Geometry: final body of the model. Coordinates: model frame, mm. A direction names the side the tool comes from. Round coordinates to 2 decimals unless told otherwise and drop trailing zeros. Loops run counter-clockwise (first coordinate to the right, second up) from the corner with the lowest first, then second, coordinate; pieces in that order, holes last. Notation, with made-up numbers: (49, 60.25) - (105, 60.25) arc R18 ccw to (105, 78.25) - close; hole circle Ø4 at (32.25, 41). An arc over 180 degrees is marked (long way). Answer as a JSON object with one key per item and string values. Group by question number.
Item 1: Section D-D (z = -8). Return the cut outline in (x, y).
Item 2: First-contact query: pin 1 (3 mm diameter, centred on y = 8.5, z = 16, fed in from +X); pin 2 (2 mm diameter, centred on x = 0.5, z = -2.5, fed in from -Y); pin 3 (2 mm diameter, centred on y = 15, z = -1, fed in from -X); pin 4 (4 mm diameter, centred on y = 4, z = 3.5, fed in from +X). Flat tips, straight axial feed; report the tip coordinate or a pass-through.
Item 3: Reachability of faces 1 (the face through (-10.06, 7.71, 16.31)), 2 (the face through (0, 0, 20.48)) from +Z, -Z, +X, -X, +Y, -Y: full face, straight path, thin tool, end or side. Return the list, or none.
Item 4: Line query: line 1 (Z direction, x = -17, y = 0.5); line 2 (Z direction, x = 8, y = -9); line 3 (X direction, y = -6, z = 5). Output: solid intervals per line, ascending.
Item 5: Draft query along Z for faces 3 (the face through (2.7, -14.2, -4.92)), 4 (the face through (-8.87, 6.8, 10.67)), 5 (the face through (-10.06, 7.71, 1.72)). Return one class per face: released by +Z, released by -Z, zero draft, split by the parting line, or undercut.
Item 6: Section C-C (z = 3). Return the cut outline in (x, y), plus the area to 3 significant figures.
```python
from build123d import *

# Parameters (mm, degrees)
F2_SIZE = 2.54
F3_R    = 1.5875


with BuildPart() as f1:
    # F0 (on Front) → F1 (revolve)
    with BuildSketch(Plane.XZ):
        with BuildLine():
            Line((12.6746, 20.479507), (0, 20.479507))
            Line((0, 20.479507), (0, -14.699493))
            Line((0, -14.699493), (19.05, -14.699493))
            Line((19.05, -14.699493), (19.05, -4.920493))
            Line((19.05, -4.920493), (14.2621, -4.920493))
            ThreePointArc((14.2621, -4.920493), (13.139568, -4.455525), (12.6746, -3.332993))
            Line((12.6746, -3.332993), (12.6746, 6.636507))
            Line((12.6746, 6.636507), (12.6746, 6.638998))
            ThreePointArc((12.6746, 6.638998), (11.609965, 7.133359), (11.176, 8.224007))
            Line((11.176, 8.224007), (11.176, 13.050007))
            ThreePointArc((11.176, 13.050007), (11.609965, 14.140656), (12.6746, 14.635016))
            Line((12.6746, 14.635016), (12.6746, 14.637507))
            Line((12.6746, 14.637507), (12.6746, 20.479507))
        make_face()
    revolve(axis=Axis((0, 0, 2.082966), (0, 0, -1)))

    # F2
    f2_edges = [f1.edges().sort_by_distance(p)[0] for p in [
        (-12.6746, 0, 20.479507),
    ]]
    chamfer(f2_edges, length=F2_SIZE)

    # F3
    f3_edges = [f1.edges().sort_by_distance(p)[0] for p in [
        (-19.05, 0, -14.699493),
    ]]
    fillet(f3_edges, radius=F3_R)


solid = f1.part
```
Values:
{
 "1": {"outline": "circle Ø38.1 at (0, 0)"},
 "2": {"pin 1": "stops at x = 10.57", "pin 2": "stops at y = -12.68", "pin 3": "passes through", "pin 4": "stops at x = 12.52"},
 "3": {"face 1": "+Z", "face 2": "+Z, +X, -X, +Y, -Y"},
 "4": {"line 1": "z = -14.7 to -4.92", "line 2": "z = -14.7 to 6.81, 14.46 to 18.57", "line 3": "x = -11.16 to 11.16"},
 "5": {"face 3": "released by +Z", "face 4": "undercut", "face 5": "zero draft"},
 "6": {"outline": "circle Ø25.35 at (0, 0)", "area": "505 mm^2"}
}
